```python
from build123d import *

# Parameters (mm, degrees)
SALIENTE_EXTRUIR1_DEPTH = 6


with BuildPart() as part:
    # Croquis3 → Saliente-Extruir1 (new body, symmetric)
    with BuildSketch(Plane.XY.offset(3)):
        with BuildLine():
            Line((-366.794500886, -8.207293434), (-353.852479494, 23.855275987))
            ThreePointArc((-353.852479494, 23.855275987), (-358.075670455, 33.755718434), (-367.963857344, 29.503911452))
            Line((-367.963857344, 29.503911452), (-380.720202712, -2.63298212))
            ThreePointArc((-380.720202712, -2.63298212), (-376.536458173, -12.362880034), (-366.794500886, -8.207293434))
        make_face()
        with BuildLine():
            Line((-366.569674973, 28.950507876), (-379.326020341, -3.186385696))
            ThreePointArc((-379.326020341, -3.186385696), (-375.979024711, -10.970304027), (-368.185458881, -7.645834747))
            Line((-368.185458881, -7.645834747), (-355.243437488, 24.416734674))
            ThreePointArc((-355.243437488, 24.416734674), (-358.633103918, 32.363142427), (-366.569674973, 28.950507876))
        make_face(mode=Mode.SUBTRACT)
    extrude(amount=SALIENTE_EXTRUIR1_DEPTH, both=True)


solid = part.part
```
Geometry check sheet. Reference: the model listing, model coordinates, mm. A direction names the side the tool comes from. Round coordinates to 2 decimals unless told otherwise and drop trailing zeros. Write each loop counter-clockwise with the first axis right and the second up, starting at its lowest first coordinate (ties: lowest second). Pieces come first, ordered by that corner, then holes. Notation, with made-up numbers: (27.5, 87) - (82.5, 87) arc R25 cw to (82.5, 109) - close; hole circle Ø7 at (-4, -26). An arc over 180 degrees is marked (long way). Write each question's results on one line, items separated by ' | '.
(1) Thickness scan on probe 1 along X at (y, z) = (-1, 7); probe 2 along X at (y, z) = (-6, 1.5); probe 3 along Y at (x, z) = (-358.5, -1.25). Record the ranges inside material, lowest first. Write a range as from..to.
Computed:
probe 1: x = -380.07..-378.46, -365.5..-363.89 | probe 2: x = -381.23..-379.72, -367.52..-365.9 | probe 3: y = 12.34..16.35, 32.31..33.91
(2) Set-up check for faces 1 (the face through (-360.414, 7.6, 3.084)), 2 (the face through (-361.805, 8.161, 3.084)): record each of +Z, -Z, +X, -X, +Y, -Y from which the full face is reachable in a straight line by a thin tool's end or side.
Computed:
face 1: +Z, -Z, +X, -Y | face 2: +Z, -Z
(3) Depth check by flat-ended pin: pin 1 Ø6 at (x, z) = (-368, 6) entering from +Y; pin 2 Ø1 at (y, z) = (1, -0.5) entering from -X; pin 3 Ø1.5 at (x, y) = (-363, 8.5) entering from -Z; pin 4 Ø5 at (x, z) = (-368.5, 4.5) entering from -Y. Enter the tip coordinate at first touch or a pass-through.
Computed:
pin 1: stops at y = 33.1 | pin 2: stops at x = -379.48 | pin 3: passes through | pin 4: stops at y = -12.38
(4) Sectioned sample at B-B, the plane y = -5.4. Enter the section's corners in (x, z), plus the area to 3 significant figures.
Computed:
outline: (-381.25, -3) - (-379.75, -3) - (-379.75, 9) - (-381.25, 9) - close; (-367.28, -3) - (-365.66, -3) - (-365.66, 9) - (-367.28, 9) - close | area: 37.4 mm^2
(5) Draft check along X on faces 3 (the face through (-372.859, 13.107, 3.084)), 4 (the face through (-374.253, 13.66, 3.084)), 5 (the face through (-374, 13, 9)). Enter one of: pulls with the +X half, pulls with the -X half, needs draft (parallel to the pull), parting line crosses it, or undercut.
Computed:
face 3: undercut | face 4: pulls with the -X half | face 5: needs draft
(6) Sectioned sample at C-C, the plane x = -358. Enter the section's corners in (y, z), plus the area to 3 significant figures.
Computed:
outline: (13.58, -3) - (17.59, -3) - (17.59, 9) - (13.58, 9) - close; (32.07, -3) - (33.72, -3) - (33.72, 9) - (32.07, 9) - close | area: 68.0 mm^2
